The listing builds one solid part. Answer for the finished solid, in the listing's coordinates (mm). Face numbers are marked on the shaded views. A direction names the side the tool comes from. Coordinates: 2 decimals unless noted, no trailing zeros. Order: outer loops, then holes, each group sorted by start corner. A loop starts at its lowest first (then second) coordinate and runs counter-clockwise, first axis right, second up. Notation, with made-up numbers: (32.5, 14.5) -> (90.5, 14.5) arc R18 cw to (90.5, 18.5) -> close; hole circle Ø4 at (30.25, 19). An arc over 180 degrees is marked (long way). Return JSON: item names as keys, results as strings.
```python
from build123d import *

# Parameters (mm, degrees)
SKETCH1_R           = 4.7625
SKETCH1_R_2         = 4
SKETCH1_R_3         = 3.175
BOSS_EXTRUDE1_DEPTH = 12.7
BOSS_EXTRUDE2_DEPTH = 1.27
SKETCH1_6_R         = 3.175
CUT_EXTRUDE1_DEPTH  = 6.477
SKETCH1_10_R        = 4
CUT_EXTRUDE3_DEPTH  = 8.89
FILLET1_R           = 3.81
FILLET3_R           = 3.81
FILLET4_R           = 3.175
FILLET5_R           = 7.62


with BuildPart() as part:
    # Sketch1 → Boss-Extrude1 (new body)
    with BuildSketch(Plane(origin=(0, 0, 0), x_dir=(0, 1, 0), z_dir=(0, 0, 1))):
        with BuildLine():
            Line((-26.499431941, 0.950631657), (-2.449998994, -7.215393609))
            ThreePointArc((-2.449998994, -7.215393609), (3.866048142, -6.56643524), (7.497932311, -1.358459074))
            Line((7.497932311, -1.358459074), (16.069122988, 45.94970705))
            ThreePointArc((16.069122988, 45.94970705), (19.672222889, 55.119231342), (26.493389209, 62.227972063))
            Line((26.493389209, 62.227972063), (35.774163974, 68.726440514))
            ThreePointArc((35.774163974, 68.726440514), (38.958321373, 75.962988676), (34.009705021, 82.128836862))
            Line((34.009705021, 82.128836862), (16.544511529, 88.485647429))
            Line((16.544511529, 88.485647429), (-10.358349656, 77.508379092))
            Line((-10.358349656, 77.508379092), (-30.779024566, 42.987968953))
            ThreePointArc((-30.779024566, 42.987968953), (-31.601546647, 36.844959103), (-27.757349656, 31.983348043))
            Line((-27.757349656, 31.983348043), (-27.757349656, 15.42998529))
            ThreePointArc((-27.757349656, 15.42998529), (-31.855063811, 7.779670964), (-26.499431941, 0.950631657))
        make_face()
        with Locations(Location((0, 0, 0), (0, 0, 270))):
            Circle(SKETCH1_R, mode=Mode.SUBTRACT)
        with Locations(Location((31.403511529, 74.968379092, 0), (0, 0, 270))):
            Circle(SKETCH1_R_2, mode=Mode.SUBTRACT)
        with Locations(Location((-23.947349656, 38.946666667, 0), (0, 0, 270))):
            Circle(SKETCH1_R_3, mode=Mode.SUBTRACT)
        with Locations(Location((-23.947349656, 8.466666667, 0), (0, 0, 270))):
            Circle(SKETCH1_R_3, mode=Mode.SUBTRACT)
        with BuildLine():
            Line((-9.469349656, 47.836666667), (-9.469349656, 11.917365883))
            ThreePointArc((-9.469349656, 11.917365883), (-7.295140555, 7.750499045), (-2.633609794, 7.15041953))
            ThreePointArc((-2.633609794, 7.15041953), (-1.656512431, 7.437766235), (-0.649822418, 7.592241489))
            ThreePointArc((-0.649822418, 7.592241489), (4.576435948, 9.875722251), (7.339639123, 14.86498764))
            Line((7.339639123, 14.86498764), (12.10584978, 41.171797748))
            ThreePointArc((12.10584978, 41.171797748), (10.181808987, 48.455026751), (3.358262084, 51.646666667))
            Line((3.358262084, 51.646666667), (-5.659349656, 51.646666667))
            ThreePointArc((-5.659349656, 51.646666667), (-8.353426493, 50.530743503), (-9.469349656, 47.836666667))
        make_face(mode=Mode.SUBTRACT)
    extrude(amount=BOSS_EXTRUDE1_DEPTH)

    # Sketch1<4> → Boss-Extrude2 (add)
    with BuildSketch(Plane(origin=(0, 0, 0), x_dir=(0, 1, 0), z_dir=(0, 0, 1))):
        with BuildLine():
            ThreePointArc((-5.659349656, 51.646666667), (-8.353426493, 50.530743503), (-9.469349656, 47.836666667))
            Line((-9.469349656, 47.836666667), (-9.469349656, 11.917365883))
            ThreePointArc((-9.469349656, 11.917365883), (-7.295140555, 7.750499045), (-2.633609794, 7.15041953))
            ThreePointArc((-2.633609794, 7.15041953), (-1.656512431, 7.437766235), (-0.649822418, 7.592241489))
            ThreePointArc((-0.649822418, 7.592241489), (4.576435948, 9.875722251), (7.339639123, 14.86498764))
            Line((7.339639123, 14.86498764), (12.10584978, 41.171797748))
            ThreePointArc((12.10584978, 41.171797748), (10.181808987, 48.455026751), (3.358262084, 51.646666667))
            Line((3.358262084, 51.646666667), (-5.659349656, 51.646666667))
        make_face()
    extrude(amount=BOSS_EXTRUDE2_DEPTH)

    # Sketch1<6> → Cut-Extrude1 (cut)
    with BuildSketch(Plane(origin=(0, 0, 0), x_dir=(0, 1, 0), z_dir=(0, 0, 1))):
        with BuildLine():
            ThreePointArc((-27.757349656, 15.42998529), (-31.855063811, 7.779670964), (-26.499431941, 0.950631657))
            Line((-26.499431941, 0.950631657), (-11.247349656, -4.228238446))
            Line((-11.247349656, -4.228238446), (-11.247349656, 51.646666667))
            Line((-11.247349656, 51.646666667), (-25.656940256, 51.646666667))
            Line((-25.656940256, 51.646666667), (-30.779024566, 42.987968953))
            ThreePointArc((-30.779024566, 42.987968953), (-31.601546647, 36.844959103), (-27.757349656, 31.983348043))
            Line((-27.757349656, 31.983348043), (-27.757349656, 15.42998529))
        make_face()
        with Locations(Location((-23.947349656, 8.466666667, 0), (0, 0, 270))):
            Circle(SKETCH1_6_R, mode=Mode.SUBTRACT)
        with Locations(Location((-23.947349656, 38.946666667, 0), (0, 0, 270))):
            Circle(SKETCH1_6_R, mode=Mode.SUBTRACT)
    extrude(amount=CUT_EXTRUDE1_DEPTH, mode=Mode.SUBTRACT)

    # Sketch1<10> → Cut-Extrude3 (cut)
    # profile 1 of 3: a face of its own
    with BuildSketch(Plane(origin=(0, 0, 0), x_dir=(0, 1, 0), z_dir=(0, 0, 1))):
        with BuildLine():
            Line((17.433511529, 88.162077891), (17.433511529, 50.740503147))
            ThreePointArc((17.433511529, 50.740503147), (21.118462359, 57.150658387), (26.493389209, 62.227972063))
            Line((26.493389209, 62.227972063), (35.774163974, 68.726440514))
            ThreePointArc((35.774163974, 68.726440514), (38.958321373, 75.962988676), (34.009705021, 82.128836862))
            Line((34.009705021, 82.128836862), (17.433511529, 88.162077891))
        make_face()
        with Locations(Location((31.403511529, 74.968379092, 0), (0, 0, 270))):
            Circle(SKETCH1_10_R, mode=Mode.SUBTRACT)
    # profile 2 of 3: a face of its own
    with BuildSketch(Plane(origin=(0, 0, 0), x_dir=(0, 1, 0), z_dir=(0, 0, 1))):
        Polygon((-11.247349656, 76.005556842), (-24.605157851, 53.424666667), (-11.247349656, 53.424666667), align=None)
    # profile 3 of 3: a face of its own
    with BuildSketch(Plane(origin=(0, 0, 0), x_dir=(0, 1, 0), z_dir=(0, 0, 1))):
        Polygon((15.655511529, 88.122905656), (-9.469349656, 77.871120864), (-9.469349656, 53.424666667), (15.655511529, 53.424666667), align=None)
    extrude(amount=CUT_EXTRUDE3_DEPTH, mode=Mode.SUBTRACT)

    # Mirror1: part across face


with BuildPart() as part_1:
    add(part.part)
    add(part.part.mirror(Plane(origin=(-30.744300958, 0.707665305, 0), x_dir=(1, 0, 0), z_dir=(0, 0, -1))))

    # Fillet1
    fillet1_edges = [part_1.edges().sort_by_distance(p)[0] for p in [
        (-69.451290519, 17.433511529, 8.89),
        (-51.646666667, -18.452144956, 6.477),
        (-51.646666667, -18.452144956, -6.477),
        (-53.424666667, -17.926253754, 8.89),
        (-53.424666667, -17.926253754, -8.89),
        (-70.773786162, 15.655511529, 8.89),
        (-65.647893765, -9.469349656, 8.89),
        (-65.647893765, -9.469349656, -8.89),
        (-70.773786162, 15.655511529, -8.89),
        (-69.451290519, 17.433511529, -8.89),
    ]]
    fillet(fillet1_edges, radius=FILLET1_R)

    # Fillet3
    # the kernel refuses this fillet: 3.81 mm, written as the material it takes off along each edge
    with BuildSketch(Plane(origin=(-77.508379092, -10.358349656, -15.90517458), x_dir=(-0.3777939966211631, 0.9258896781566412, 0), z_dir=(0, 0, 1))) as fillet3_piece_1:
        with BuildLine():
            CenterArc((FILLET3_R * 0.336501268256, -FILLET3_R), FILLET3_R, 90, 37.196303294)
            Line((-FILLET3_R * 0.268046453486, -FILLET3_R * 0.203431075087), (0, 0))
            Line((0, 0), (FILLET3_R * 0.336501268256, 0))
        make_face()
    extrude(amount=31.81034916, mode=Mode.SUBTRACT)
    with BuildSketch(Plane(origin=(-88.485647429, 16.544511529, -16.375115103), x_dir=(0.3420201433256622, 0.9396926207859108, 0), z_dir=(0, 0, 1))) as fillet3_piece_2:
        with BuildLine():
            CenterArc((FILLET3_R * 0.385838855973, -FILLET3_R), FILLET3_R, 90, 42.197104506)
            Line((-FILLET3_R * 0.285844295256, -FILLET3_R * 0.259161458646), (0, 0))
            Line((0, 0), (FILLET3_R * 0.385838855973, 0))
        make_face()
    extrude(amount=32.750230206, mode=Mode.SUBTRACT)

    # Fillet4
    fillet4_edges = [part_1.edges().sort_by_distance(p)[0] for p in [
        (-53.424666667, -11.247349656, 0),
        (-66.620111754, -11.247349656, -8.89),
        (-66.620111754, -11.247349656, 8.89),
        (-54.54058983, -11.247349656, -7.774076836),
        (-54.54058983, -11.247349656, 7.774076836),
        (-21.80421411, -11.247349656, 6.477),
        (-51.646666667, -11.247349656, 0),
        (-21.80421411, -11.247349656, -6.477),
        (-50.530743503, -11.247349656, -5.361076836),
        (-50.530743503, -11.247349656, 5.361076836),
    ]]
    fillet(fillet4_edges, radius=FILLET4_R)

    # Fillet5
    fillet5_edges = [part_1.edges().sort_by_distance(p)[0] for p in [
        (-31.983348043, -27.757349656, -9.5885),
        (-15.42998529, -27.757349656, -9.5885),
        (-15.42998529, -27.757349656, 9.5885),
        (-31.983348043, -27.757349656, 9.5885),
    ]]
    fillet(fillet5_edges, radius=FILLET5_R)


solid = part_1.part
```
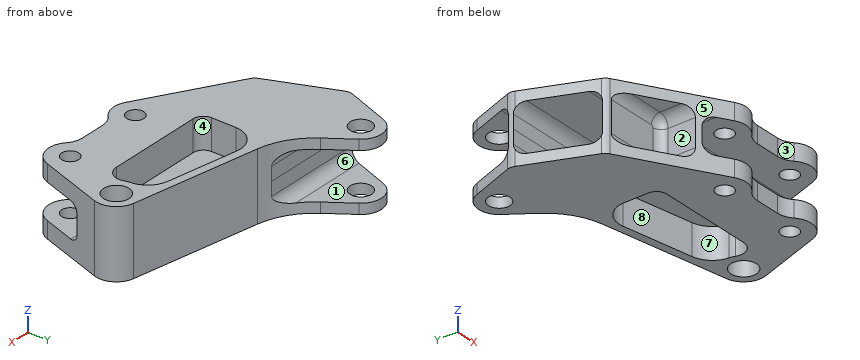
Item 1: Find the intervals of material crossed by probe 1 along Y at (x, z) = (-65, 4.5); probe 2 along Z at (x, y) = (-81, -1); probe 3 along Z at (x, y) = (-14, 3), in increasing order.
Answer list:
{"probe 1": "-11.25 to -9.47, 15.66 to 17.43", "probe 2": "-12.7 to -8.89, 8.89 to 12.7", "probe 3": "-1.27 to 1.27"}
Item 2: Flat-ended cylindrical pins translate along their axes: pin 1 (2.5 mm diameter, centred on x = -72.5, z = -3, fed in from -Y); pin 2 (5 mm diameter, centred on x = -65.5, z = -0.5, fed in from +Y); pin 3 (3 mm diameter, centred on y = 10, z = 5.5, fed in from -X). Find the tip coordinate at first contact, or state that the pin passes through.
Answer list:
{"pin 1": "y = -11.25", "pin 2": "y = 17.43", "pin 3": "x = -53.42"}
Item 3: The part is cut by section A-A on x = -39. Determine the outline of the cut face in (y, z) (3 decimals), plus the area to 3 significant figures.
Answer list:
{"outline": "(-31.885, -12.7) -> (-27.122, -12.7) -> (-27.122, -6.477) -> (-31.885, -6.477) -> close; (-31.885, 6.477) -> (-27.122, 6.477) -> (-27.122, 12.7) -> (-31.885, 12.7) -> close; (-20.773, -12.7) -> (-9.469, -12.7) -> (-9.469, -1.27) -> (11.712, -1.27) -> (11.712, -12.7) -> (14.81, -12.7) -> (14.81, 12.7) -> (11.712, 12.7) -> (11.712, 1.27) -> (-9.469, 1.27) -> (-9.469, 12.7) -> (-20.773, 12.7) -> (-20.773, 6.477) -> (-14.422, 6.477) arc R3.175 cw to (-11.247, 3.302) -> (-11.247, -3.302) arc R3.175 cw to (-14.422, -6.477) -> (-20.773, -6.477) -> close", "area": "360 mm2"}
Item 4: Which of the six approach directions +Z, -Z, +X, -X, +Y, -Y give full straight-line access (tool end or side, diameter ignored) to the marked faces 1, 2, 3 and 4?
Answer list:
{"face 1": "+X, -X, +Y", "face 2": "-X, -Y", "face 3": "+Z, -Z, -Y", "face 4": "+Z"}
Item 5: The part is cut by section B-B on x = -3.5. Determine the outline of the cut face in (y, z) (3 decimals), plus the area to 3 significant figures.
Answer list:
{"outline": "(-30.139, -12.7) -> (-3.23, -12.7) -> (-3.23, 12.7) -> (-30.139, 12.7) -> (-30.139, 6.477) -> (-14.422, 6.477) arc R3.175 cw to (-11.247, 3.302) -> (-11.247, -3.302) arc R3.175 cw to (-14.422, -6.477) -> (-30.139, -6.477) -> close; (3.23, -12.7) -> (8.378, -12.7) -> (8.378, 12.7) -> (3.23, 12.7) -> close", "area": "574 mm2"}
Item 6: Determine the mould class of the marked faces 5, 6, 7 and 8 for opening direction X: pulls with the +X half, pulls with the -X half, needs draft (parallel to the pull), parting line crosses it, or undercut.
Answer list:
{"face 5": "pulls with the -X half", "face 6": "needs draft", "face 7": "undercut", "face 8": "undercut"}
Item 7: The part is cut by section C-C on x = -27. Determine the outline of the cut face in (y, z) (3 decimals), plus the area to 3 significant figures.
Answer list:
{"outline": "(-27.757, -12.7) -> (-9.469, -12.7) -> (-9.469, -1.27) -> (9.538, -1.27) -> (9.538, -12.7) -> (12.636, -12.7) -> (12.636, 12.7) -> (9.538, 12.7) -> (9.538, 1.27) -> (-9.469, 1.27) -> (-9.469, 12.7) -> (-27.757, 12.7) -> (-27.757, 6.477) -> (-14.422, 6.477) arc R3.175 cw to (-11.247, 3.302) -> (-11.247, -3.302) arc R3.175 cw to (-14.422, -6.477) -> (-27.757, -6.477) -> close", "area": "382 mm2"}
